Study the drawing (mm; zero at the part's minimum x, y, z) and answer. Give positions to 0.01 mm unless a question says otherwise; leave off trailing zeros. Write each loop counter-clockwise with the first axis right and the second up, starting at its lowest first coordinate (ties: lowest second). Pieces come first, ordered by that corner, then holes. Notation, with made-up numbers: (32, 33.25) -> (50, 33.25) arc R22 ccw to (50, 64.25) -> close; hole circle Ø3 at (-34, -16.75). An arc over 180 degrees is marked (long way). Use CSV: the item, a comma, the result in double quotes. Start each with the question number.
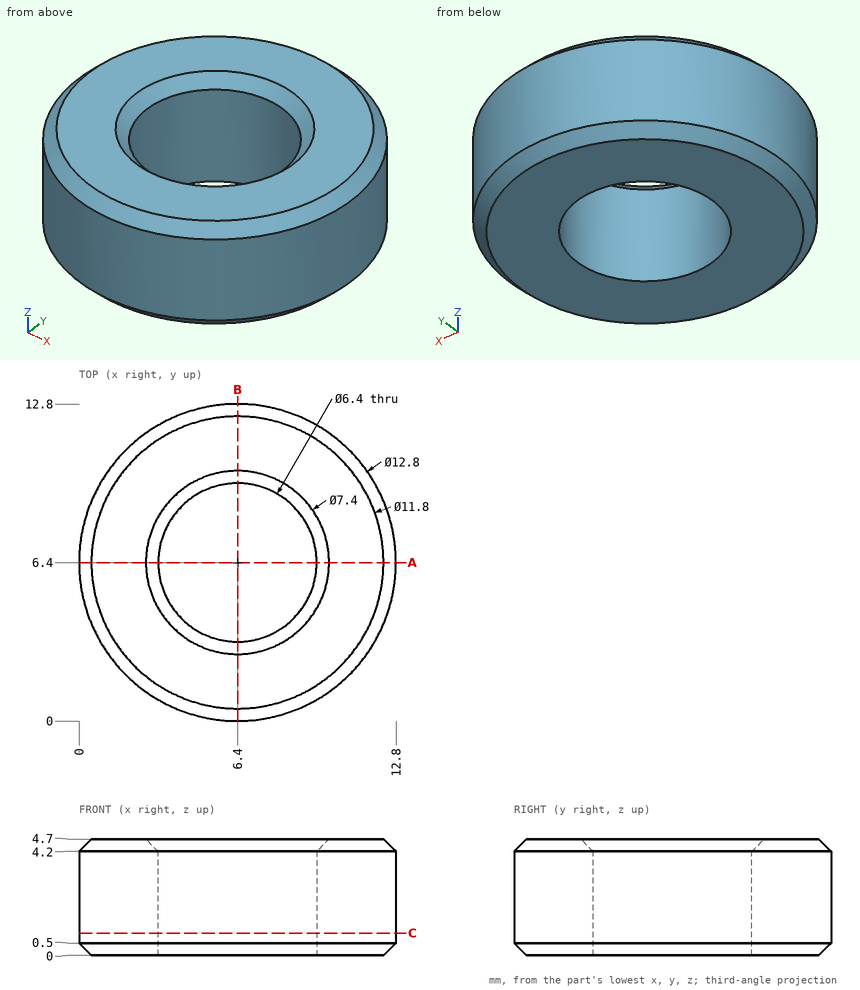
Q1. Straight lines are drawn through the part: L1, parallel to Y at x = 6.4, z = 2.7; L2, parallel to X at y = 5.25, z = 2.75; L3, parallel to Y at x = 9, z = 1.95. For each, find the intervals that lie inside material, in ascending order.
Q2. Section C-C on z = 0.9 is taken. Give the vertices of the cut face in (x, y).
Q3. Flat-ended cylindrical pins translate along their axes: pin 1 Ø1.5 at (x, z) = (10.5, 1) entering from -Y; pin 2 Ø6 at (x, y) = (6.4, 6.4) entering from -Z. Find the tip coordinate at first contact, or state that the pin passes through.
Q4. Section A-A on y = 6.4 is taken. Give the vertices of the cut face in (x, z), then the cut area to 3 significant figures.
Output:
1,L1,"0 to 3.2, 9.6 to 12.8"
1,L2,"0.1 to 3.41, 9.39 to 12.7"
1,L3,"0.55 to 4.53, 8.27 to 12.25"
2,outline,"circle Ø12.8 at (6.4, 6.4); hole circle Ø6.4 at (6.4, 6.4)"
3,pin 1,"y = 0.95"
3,pin 2,"through"
4,outline,"(0, 0.5) -> (0.5, 0) -> (3.2, 0) -> (3.2, 4.2) -> (2.7, 4.7) -> (0.5, 4.7) -> (0, 4.2) -> close; (9.6, 0) -> (12.3, 0) -> (12.8, 0.5) -> (12.8, 4.2) -> (12.3, 4.7) -> (10.1, 4.7) -> (9.6, 4.2) -> close"
4,area,"29.3 mm²"
